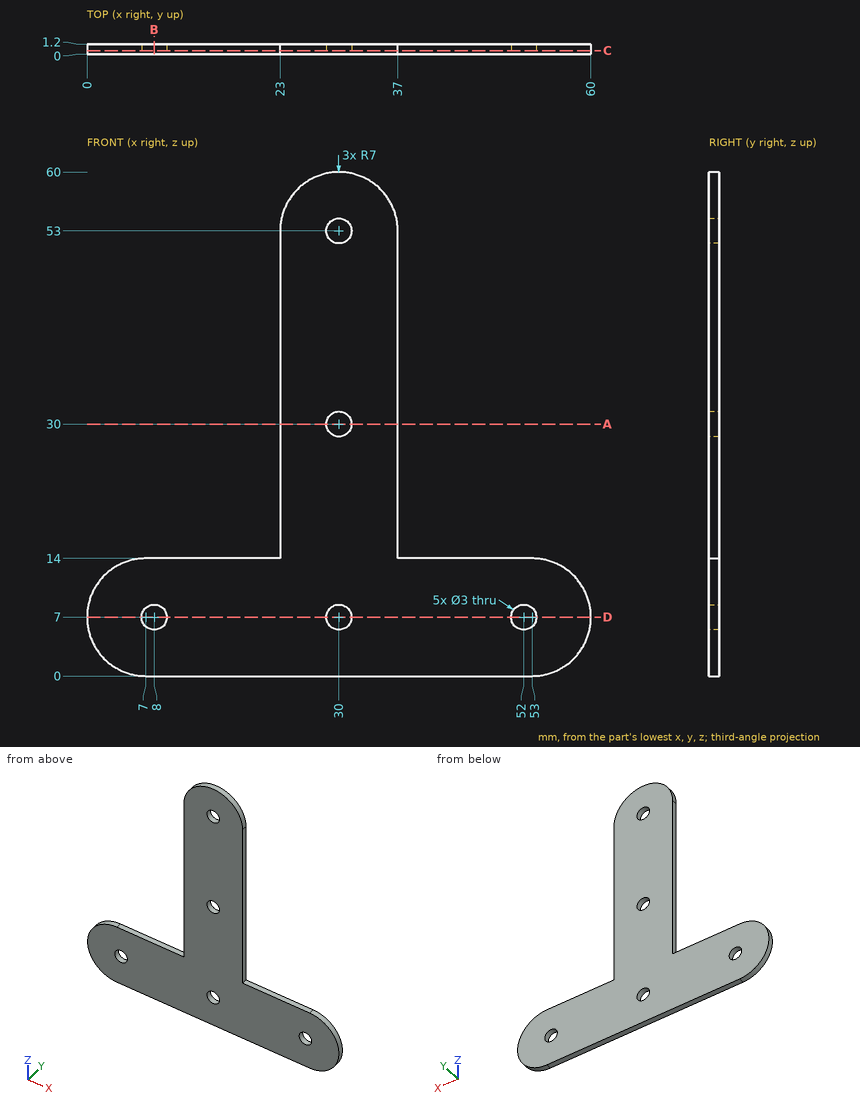
Part print with two shaded views. Sizes in mm from the minimum x, y, z corner. Round coordinates to 2 decimals unless told otherwise and drop trailing zeros. Write each loop counter-clockwise with the first axis right and the second up, starting at its lowest first coordinate (ties: lowest second). Pieces come first, ordered by that corner, then holes. Notation, with made-up numbers: M -6.5,-25.5 L 10.5,-25.5 A19 cw 10.5,9.5 Z; hole C 48,39 d6. An arc over 180 degrees is marked long. Use CSV: the item, a comma, the result in double quotes.
1. Saw through at C-C (y = 0.4). Give the cut face in (x, z), plus the area to 3 significant figures.
Reply:
outline,"M 7,0 L 53,0 A7 ccw 53,14 L 37,14 L 37,53 A7 ccw 23,53 L 23,14 L 7,14 A7 ccw Z; hole C 8,7 d3; hole C 30,7 d3; hole C 30,30 d3; hole C 30,53 d3; hole C 52,7 d3"
area,"1,390 mm²"
2. Saw through at B-B (x = 8). Give the cut face in (y, z), plus the area to 3 significant figures.
Reply:
outline,"M 0,0 L 1.2,0 L 1.2,5.5 L 0,5.5 Z; M 0,8.5 L 1.2,8.5 L 1.2,14 L 0,14 Z"
area,"13.2 mm²"
3. Flat gauge pins, fed straight in: pin 1 (0.6 mm diameter, centred on x = 13.5, y = 0.5, fed in from +Z); pin 2 (1.8 mm diameter, centred on x = 30, z = 30, fed in from +Y) (3 decimals); pin 3 (5 mm diameter, centred on x = 52, z = 7, fed in from +Y). Where does each tip first touch, or does it go through?
Reply:
pin 1,"stops at z = 14"
pin 2,"passes through"
pin 3,"stops at y = 1.2"
4. Wall check: probe 1 along X at (y, z) = (0.9, 7); probe 2 along X at (y, z) = (0.35, 53); probe 3 along X at (y, z) = (1.1, 6.5). Give the ranges that are in metal, low to high. Write a range as from..to.
Reply:
probe 1,"x = 0..6.5, 9.5..28.5, 31.5..50.5, 53.5..60"
probe 2,"x = 23..28.5, 31.5..37"
probe 3,"x = 0.02..6.59, 9.41..28.59, 31.41..50.59, 53.41..59.98"
5. Saw through at A-A (z = 30). Give the cut face in (x, y).
Reply:
outline,"M 23,0 L 28.5,0 L 28.5,1.2 L 23,1.2 Z; M 31.5,0 L 37,0 L 37,1.2 L 31.5,1.2 Z"
6. Saw through at D-D (z = 7). Give the cut face in (x, y).
Reply:
outline,"M 0,0 L 6.5,0 L 6.5,1.2 L 0,1.2 Z; M 9.5,0 L 28.5,0 L 28.5,1.2 L 9.5,1.2 Z; M 31.5,0 L 50.5,0 L 50.5,1.2 L 31.5,1.2 Z; M 53.5,0 L 60,0 L 60,1.2 L 53.5,1.2 Z"
